Can you work these out from the drawing? Everything is in mm from the part's minimum corner. Coordinates: 2 decimals unless noted, no trailing zeros. Write each loop counter-clockwise with the first axis right and the second up, starting at its lowest first coordinate (ties: lowest second). Pieces come first, ordered by that corner, then holes. Notation, with made-up numbers: M 68,30.25 L 85,30.25 A13 cw 85,34.25 Z; hole C 1.5,83 d7. An arc over 180 degrees is marked long. Answer as a JSON object with one key per item and string values. Group by question number.
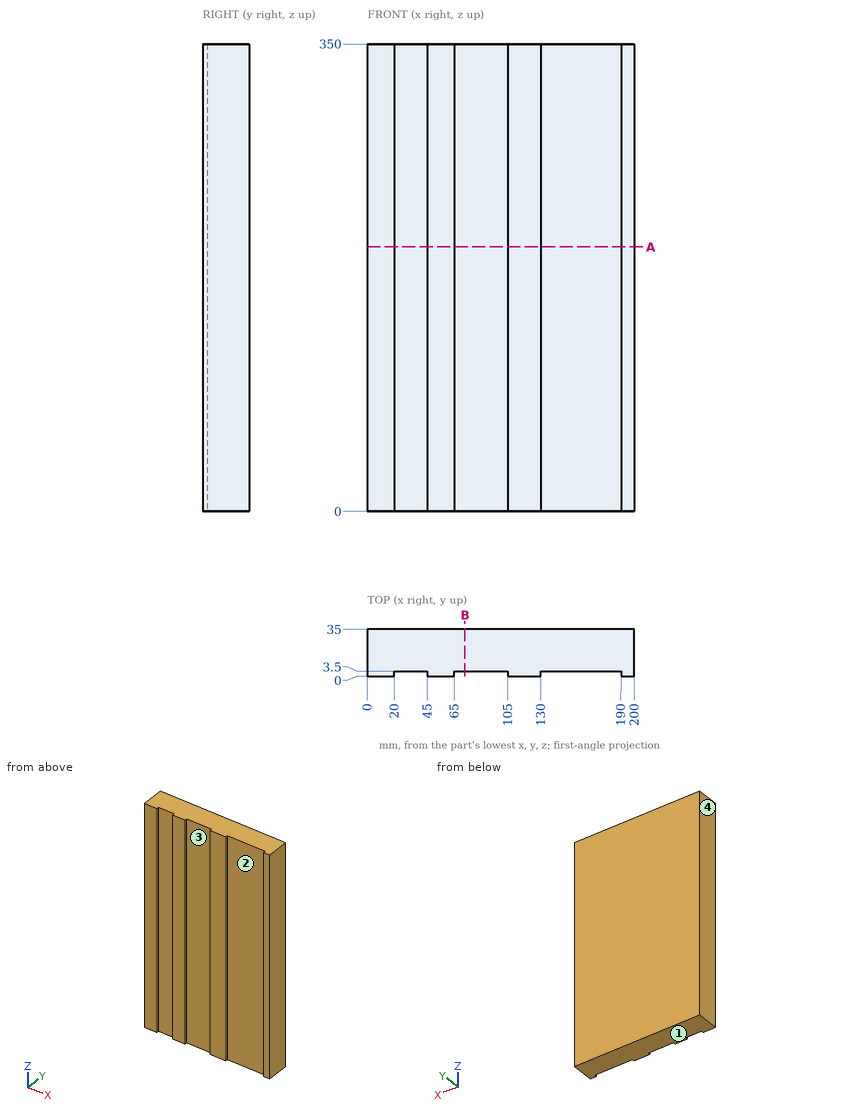
Q1. If we section it at A-A on z = 198: List the corners of the cut face in (x, y) for me, and give its area (3 significant figures).
Q2. Please list where these lines run through material, in increasing order: L1, parallel to X at y = 3, z = 334; L2, parallel to Y at x = 103, z = 194.
Q3. We'd pull the mould along X, two halves only. Please class the marked faces 1, 2, 3 and 4: pulls with the +X half, pulls with the -X half, needs draft (parallel to the pull), parting line crosses it, or undercut.
Q4. If we section it at B-B on x = 73: List the corners of the cut face in (y, z) for me.
Reply:
{
 "1": {"outline": "M 0,0 L 20,0 L 20,3.5 L 45,3.5 L 45,0 L 65,0 L 65,3.5 L 105,3.5 L 105,0 L 130,0 L 130,3.5 L 190,3.5 L 190,0 L 200,0 L 200,35 L 0,35 Z", "area": "6,560 mm^2"},
 "2": {"L1": "0 to 20, 45 to 65, 105 to 130, 190 to 200", "L2": "3.5 to 35"},
 "3": {"face 1": "needs draft", "face 2": "undercut", "face 3": "undercut", "face 4": "pulls with the -X half"},
 "4": {"outline": "M 3.5,0 L 35,0 L 35,350 L 3.5,350 Z"}
}
